```python
from build123d import *

# Parameters (mm, degrees)
SKETCH1_R           = 2.25
BOSS_EXTRUDE1_DEPTH = 2


with BuildPart() as part:
    # Sketch1 → Boss-Extrude1 (new body)
    with BuildSketch(Plane.XY):
        with BuildLine():
            ThreePointArc((-65.072201119, -14.494287215), (-60.59129068, -32.898192856), (-76.810886122, -42.68118958))
            Line((-76.810886122, -42.68118958), (-191.898124009, -58.394928446))
            Line((-191.898124009, -58.394928446), (-191.898124009, -58.897796779))
            Line((-191.898124009, -58.897796779), (-191.898124009, -136.379261887))
            ThreePointArc((-191.898124009, -136.379261887), (-66.915619532, -186.523885549), (52.083721608, -123.48210166))
            Line((52.083721608, -123.48210166), (52.083721608, -50.984586674))
            Line((52.083721608, -50.984586674), (37.834963232, -37.825461025))
            ThreePointArc((37.834963232, -37.825461025), (14.189227202, -36.712872143), (17.530284751, -13.277940505))
            Line((17.530284751, -13.277940505), (17.466018163, 14.941165213))
            Line((17.466018163, 14.941165213), (-17.533981861, 14.861463987))
            Line((-17.533981861, 14.861463987), (-17.442886515, -25.137999382))
            Line((-17.442886515, -25.137999382), (-17.442885293, -25.138536013))
            add(Edge.make_bspline(
                [(-64.623988745, -14.046074897), (-63.208317509, -14.654705213), (-59.235254763, -16.288548622), (-52.683559955, -18.641296662), (-44.896066709, -20.933273776), (-33.264108999, -23.619131202), (-24.061605806, -24.778728303), (-17.442885293, -25.138536013)],
                knots=[0.054790311, 0.054790311, 0.054790311, 0.054790311, 0.119867337, 0.236316132, 0.352764926, 0.46921372, 0.751953645, 0.751953645, 0.751953645, 0.751953645], degree=3))
            Line((-64.623988745, -14.046074897), (-65.072201119, -14.494287215))
        make_face()
        with Locations((-25.361610976, -39.621277184)):
            Circle(SKETCH1_R, mode=Mode.SUBTRACT)
        with Locations((-25.361610976, -31.831277184)):
            Circle(SKETCH1_R, mode=Mode.SUBTRACT)
    extrude(amount=BOSS_EXTRUDE1_DEPTH)


solid = part.part
```
CAD build for the part. Positions are in the model's coordinates, mm. Round coordinates to 2 decimals unless told otherwise and drop trailing zeros. Order: outer loops, then holes, each group sorted by start corner. A loop starts at its lowest first (then second) coordinate and runs counter-clockwise, first axis right, second up.
Item 1: Saw through at A-A on z = 1.15. State how many separate pieces and enclosed holes the cut face has, then the cut area to 3 significant figures.
Item 2: Probe line 1 along Y through (x, z) = (15, 1.4); line 2 along X through (y, z) = (3, 1); line 3 along X through (y, z) = (-32, 1.1). List the from-to ranges inside material, lowest first.
Item 3: Pin check, flat tip, straight feed: pin 1 (2.5 mm diameter, centred on x = -25.36, y = -39.62, fed in from +Z) (3 decimals). Stop position of the tip, or through.
Item 4: Saw through at C-C on x = -108. Write the cut outline in (y, z).
Item 5: Mould opens along Y. For faces 1 (the face through (-68.859, -186.615, 0.986)), 2 (the face through (-72, -107, 2)), 3 (the face through (45.06, -44.5, 0.99)), 4 (the face through (14.43, -37, 0.99)) say: pulls with the +Y half, pulls with the -Y half, needs draft (parallel to the pull), parting line crosses it, or undercut.
Item 6: Saw through at B-B on y = -148. Write the cut outline in (x, z), then the cut area to 3 significant figures.
Reported:
1. separate pieces: 1
1. enclosed holes: 2
1. area: 32,800 mm2
2. line 1: y = -158.79 to -37.62, -15.41 to 14.94
2. line 2: x = -17.51 to 17.49
2. line 3: x = -60.25 to -27.61, -23.12 to 11.49
3. pin 1: passes through
4. outline: (-183.38, 0) - (-46.94, 0) - (-46.94, 2) - (-183.38, 2) - close
5. face 1: pulls with the -Y half
5. face 2: needs draft
5. face 3: pulls with the +Y half
5. face 4: undercut
6. outline: (-179.75, 0) - (29.03, 0) - (29.03, 2) - (-179.75, 2) - close
6. area: 418 mm2
